Could you check a few things on this model? Use its own coordinates, in mm. A direction names the side the tool comes from. Give positions to 0.01 mm unless a question says otherwise; leave off trailing zeros. Order: outer loops, then holes, each group sorted by start corner. A loop starts at its lowest first (then second) coordinate and runs counter-clockwise, first axis right, second up. Notation, with made-up numbers: (23, 34.25) -> (58, 34.25) arc R20 cw to (58, 38.25) -> close; hole circle Ø4 at (67.25, 87.5). An arc over 180 degrees is marked (long way). Write each question's results on one line, items separated by ' | '.
```python
from build123d import *

# Parameters (mm, degrees)
BOSS_EXTRUDE1_DEPTH = 19


with BuildPart() as part:
    # Sketch1 → Boss-Extrude1 (new body)
    with BuildSketch(Plane.XY):
        with BuildLine():
            Line((-203, 38), (-212.5, 38))
            ThreePointArc((-212.5, 38), (-216.742640687, 36.242640687), (-218.5, 32))
            Line((-218.5, 32), (-218.5, -6))
            ThreePointArc((-218.5, -6), (-216.742640687, -10.242640687), (-212.5, -12))
            Line((-212.5, -12), (-203, -12))
            ThreePointArc((-203, -12), (-197.878679656, -9.878679656), (-200, -15))
            Line((-200, -15), (-200, -59))
            ThreePointArc((-200, -59), (-197.878679656, -64.121320344), (-203, -62))
            Line((-203, -62), (-212.5, -62))
            ThreePointArc((-212.5, -62), (-216.742640687, -63.757359313), (-218.5, -68))
            Line((-218.5, -68), (-218.5, -106))
            ThreePointArc((-218.5, -106), (-216.742640687, -110.242640687), (-212.5, -112))
            Line((-212.5, -112), (-203, -112))
            ThreePointArc((-203, -112), (-197.878679656, -109.878679656), (-200, -115))
            Line((-200, -115), (-200, -155))
            ThreePointArc((-200, -155), (-197.071067812, -162.071067812), (-190, -165))
            Line((-190, -165), (190, -165))
            ThreePointArc((190, -165), (197.071067812, -162.071067812), (200, -155))
            Line((200, -155), (200, -115))
            ThreePointArc((200, -115), (197.878679656, -109.878679656), (203, -112))
            Line((203, -112), (212.5, -112))
            ThreePointArc((212.5, -112), (216.742640687, -110.242640687), (218.5, -106))
            Line((218.5, -106), (218.5, -68))
            ThreePointArc((218.5, -68), (216.742640687, -63.757359313), (212.5, -62))
            Line((212.5, -62), (203, -62))
            ThreePointArc((203, -62), (197.878679656, -64.121320344), (200, -59))
            Line((200, -59), (200, -15))
            ThreePointArc((200, -15), (197.878679656, -9.878679656), (203, -12))
            Line((203, -12), (212.5, -12))
            ThreePointArc((212.5, -12), (216.742640687, -10.242640687), (218.5, -6))
            Line((218.5, -6), (218.5, 32))
            ThreePointArc((218.5, 32), (216.742640687, 36.242640687), (212.5, 38))
            Line((212.5, 38), (203, 38))
            ThreePointArc((203, 38), (197.878679656, 35.878679656), (200, 41))
            Line((200, 41), (200, 85))
            ThreePointArc((200, 85), (197.878679656, 90.121320344), (203, 88))
            Line((203, 88), (212.5, 88))
            ThreePointArc((212.5, 88), (216.742640687, 89.757359313), (218.5, 94))
            Line((218.5, 94), (218.5, 132))
            ThreePointArc((218.5, 132), (216.742640687, 136.242640687), (212.5, 138))
            Line((212.5, 138), (203, 138))
            ThreePointArc((203, 138), (197.878679656, 135.878679656), (200, 141))
            Line((200, 141), (200, 149))
            ThreePointArc((200, 149), (198.242640687, 153.242640687), (194, 155))
            Line((194, 155), (-194, 155))
            ThreePointArc((-194, 155), (-198.242640687, 153.242640687), (-200, 149))
            Line((-200, 149), (-200, 141))
            ThreePointArc((-200, 141), (-197.878679656, 135.878679656), (-203, 138))
            Line((-203, 138), (-212.5, 138))
            ThreePointArc((-212.5, 138), (-216.742640687, 136.242640687), (-218.5, 132))
            Line((-218.5, 132), (-218.5, 94))
            ThreePointArc((-218.5, 94), (-216.742640687, 89.757359313), (-212.5, 88))
            Line((-212.5, 88), (-203, 88))
            ThreePointArc((-203, 88), (-197.878679656, 90.121320344), (-200, 85))
            Line((-200, 85), (-200, 41))
            ThreePointArc((-200, 41), (-197.878679656, 35.878679656), (-203, 38))
        make_face()
    extrude(amount=BOSS_EXTRUDE1_DEPTH)


solid = part.part
```
Q1. For faces 4 (the flat face through (-200, -135, 9)), 5 (the flat face through (208, -12, 9)), 6 (the flat face through (200, -135, 9)), which set-ups out of +Z, -Z, +X, -X, +Y, -Y let a thin tool reach every point of the face, with its end or its side?
Here are the results:
face 4: +Z, -Z, -X, -Y | face 5: +Z, -Z, +X | face 6: +Z, -Z, +X, -Y
Q2. Suppose I cut it at A-A on y = 75.5. Please give me the cut outline in (x, z).
Here are the results:
outline: (-200, 0) -> (200, 0) -> (200, 19) -> (-200, 19) -> close
Q3. I'm going to push flat-ended pins straight in: pin 1 Ø7.5 at (x, z) = (209, 13.5) entering from -Y; pin 2 Ø5.5 at (y, z) = (52.5, 7.5) entering from +X; pin 3 Ø3 at (x, z) = (-208.5, 13) entering from +Y. Where does each tip first touch, or does it pass through?
Here are the results:
pin 1: stops at y = -112 | pin 2: stops at x = 200 | pin 3: stops at y = 138
Q4. I need wall thicknesses on line 1 along X through (y, z) = (-40.5, 11); line 2 along X through (y, z) = (-65.5, 6); line 3 along Y through (x, z) = (-194.5, 3). Which ranges of each line are inside material? Lowest first, please.
Here are the results:
line 1: x = -200 to 200 | line 2: x = -217.95 to 217.95 | line 3: y = -163.93 to 154.98
Q5. Thinking about a two-plate mould opening in Y: for faces 1 (the flat face through (208, -62, 9)), 2 (the flat face through (218.5, -87, 9)), 3 (the flat face through (3, 155, 9)), which applies, +Y half, -Y half, draft (parallel to the pull), parting line (faces both ways), or undercut?
Here are the results:
face 1: undercut | face 2: draft | face 3: +Y half
